CAD build for the part. Positions are in the model's coordinates, mm. Face numbers are marked on the shaded views. Round coordinates to 2 decimals unless told otherwise and drop trailing zeros. Loops run counter-clockwise (first coordinate to the right, second up) from the corner with the lowest first, then second, coordinate; pieces in that order, holes last.
from build123d import *

# Parameters (mm, degrees)
F0_R     = 16.05
F1_DEPTH = 1
F2_R     = 16.65
F2_R_2   = 16.05
F3_DEPTH = 20


with BuildPart() as f1:
    # F0 (on Top) → F1 (new body)
    with BuildSketch(Plane.XY):
        with BuildLine():
            ThreePointArc((0, -17), (12.020815, -12.020815), (17, 0))
            ThreePointArc((17, 0), (12.020815, 12.020815), (0, 17))
            ThreePointArc((0, 17), (-17, 0), (0, -17))
        make_face()
        Circle(F0_R, mode=Mode.SUBTRACT)
        with BuildLine():
            ThreePointArc((0, 17), (12.020815, 12.020815), (17, 0))
            ThreePointArc((17, 0), (12.020815, -12.020815), (0, -17))
            Line((0, -17), (25, -17))
            Line((25, -17), (25, 17))
            Line((25, 17), (0, 17))
        make_face()
    extrude(amount=F1_DEPTH)

    # F2 (on face) → F3 (join)
    with BuildSketch(Plane.XY.offset(1)):
        Circle(F2_R)
        Circle(F2_R_2, mode=Mode.SUBTRACT)
    extrude(amount=F3_DEPTH)


solid = f1.part
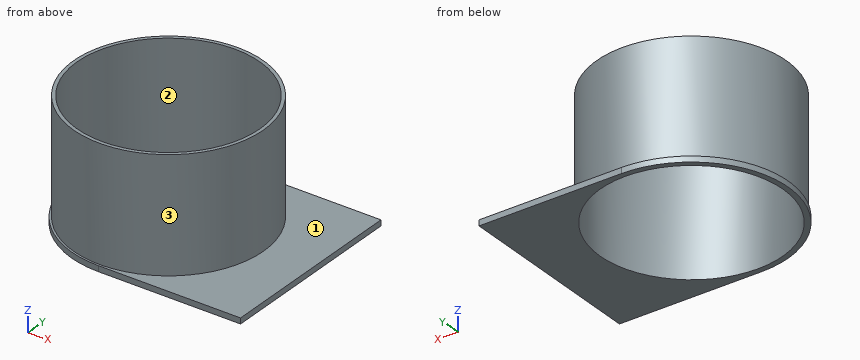
Item 1: Cut at C-C (z = 11.5). List the corners of the cut face in (x, y), plus the area to 3 significant figures.
Verdict:
outline: circle Ø33.3 at (0, 0); hole circle Ø32.1 at (0, 0)
area: 61.6 mm2
Item 2: Cut at A-A (y = 0). List the corners of the cut face in (x, z), plus the area to 3 significant figures.
Verdict:
outline: (-17, 0) - (-16.05, 0) - (-16.05, 21) - (-16.65, 21) - (-16.65, 1) - (-17, 1) - close; (16.05, 0) - (25, 0) - (25, 1) - (16.65, 1) - (16.65, 21) - (16.05, 21) - close
area: 33.9 mm2
Item 3: Flat gauge pins, fed straight in: P1, Ø8, axis at y = 9.5, z = 16.5, coming from the -X side; P2, Ø1.5, axis at y = 13, z = 12.5, coming from the -X side; P3, Ø6, axis at x = -6, z = 16.5, coming from the -Y side. Where does each tip first touch, or does it go through?
Verdict:
P1: stops at x = -15.72
P2: stops at x = -11.28
P3: stops at y = -16.38
Item 4: Cut at B-B (x = 6). List the corners of the cut face in (y, z).
Verdict:
outline: (-17, 0) - (-14.89, 0) - (-14.89, 21) - (-15.53, 21) - (-15.53, 1) - (-17, 1) - close; (14.89, 0) - (17, 0) - (17, 1) - (15.53, 1) - (15.53, 21) - (14.89, 21) - close
Item 5: Mould opens along X. For the marked faces 1, 2 and 3 say: released by +X, released by -X, zero draft, split by the parting line, or undercut.
Verdict:
face 1: zero draft
face 2: undercut
face 3: split by the parting line
Item 6: Wall check: L1, parallel to Y at x = 12.5, z = 2.75; L2, parallel to X at y = 5.5, z = 17; L3, parallel to X at y = 14, z = 15.5. Give the ranges that are in metal, low to high.
Verdict:
L1: y = -11 to -10.07, 10.07 to 11
L2: x = -15.72 to -15.08, 15.08 to 15.72
L3: x = -9.01 to -7.85, 7.85 to 9.01
